Input: part model. Units: mm. Frame: model coordinates. Face numbers are marked on the shaded views. A direction names the side the tool comes from. Round coordinates to 2 decimals unless told otherwise and drop trailing zeros. Loops run counter-clockwise (first coordinate to the right, second up) from the corner with the lowest first, then second, coordinate; pieces in that order, holes last. Notation, with made-up numbers: (-32, -10) -> (25, -10) arc R10 cw to (25, 8) -> close; hole circle Ø7 at (15, 14). An arc over 180 degrees is marked (long way). Answer as a JSON object with one key per item and string values. Group by question number.
Item 1: Section query A-A on y = 0. Return loops of the section in (x, z), and give its area (3 significant figures).
Item 2: Draft query along Z for the marked faces 1, 2, 3 and 4. Return one class per face: released by +Z, released by -Z, zero draft, split by the parting line, or undercut.
Item 3: Pin query (flat end, axial travel): pin 1 (0.9 mm diameter, centred on x = 5, y = -6, fed in from +Z); pin 2 (1.5 mm diameter, centred on x = 6.5, y = 5.5, fed in from -Z); pin 3 (3 mm diameter, centred on x = 6.5, z = -5, fed in from -Y). Return the tip coordinate at first contact, or that it passes through.
Item 4: Section query D-D on y = 3. Return loops of the section in (x, z).
Item 5: Section query C-C on x = 7.75. Return loops of the section in (y, z).
Item 6: Section query B-B on z = 0. Return loops of the section in (x, y), and give its area (3 significant figures).
Item 7: Material intervals for line 1 (Z direction, x = 2.5, y = 0); line 2 (Z direction, x = 1.75, y = 2.5), sorted ascending. Write a range as [from, to].
Item 8: Set-up query: the marked faces 5, 6 and 7. Return all of +Z, -Z, +X, -X, +Y, -Y with unobstructed straight access to the full face (end or side cutting, diameter ignored); none if empty.
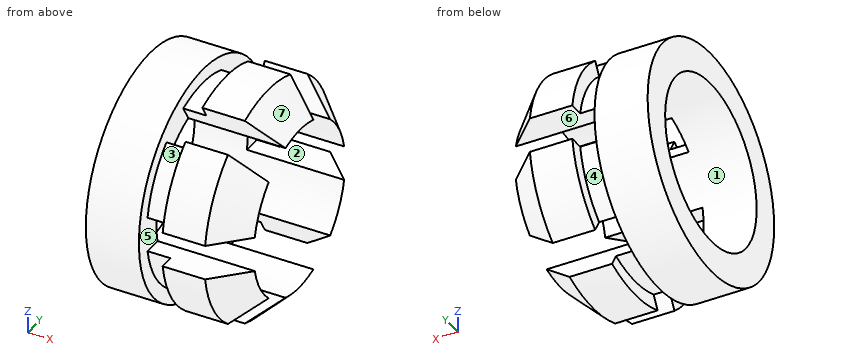
from build123d import *

# Parameters (mm, degrees)
SKETCH_1_R               = 6.5
SKETCH_1_R_2             = 4.7
EXTRUDE_1_DEPTH          = 8.5
SKETCH_2_W               = 1.3
SKETCH_2_H               = 0.8
SKETCH_4_W               = 2
SKETCH_4_H               = 13
CUT_EXTRUDE_1_DEPTH      = 8.5
PATTERN_START            = 3
PATTERN_CIRCULAR_1_DEPTH = 5.5000001


# Read off the part's stored shape, not the designer's step: Круговой массив1
with BuildPart() as part:
    # Эскиз1 → Вытянуть1 (new body)
    with BuildSketch(Plane(origin=(0, 0, 0), x_dir=(0, 0, -1), z_dir=(1, 0, 0))):
        Circle(SKETCH_1_R)
        Circle(SKETCH_1_R_2, mode=Mode.SUBTRACT)
    extrude(amount=EXTRUDE_1_DEPTH)

    # Эскиз2 → Вырез-Повернуть1 (revolve, cut)
    with BuildSketch(Plane.XY, mode=Mode.PRIVATE) as cut_revolve_1_sk:
        with Locations((3.65, 6.1)):
            Rectangle(SKETCH_2_W, SKETCH_2_H)
    revolve(cut_revolve_1_sk.sketch.rotate(Axis((8.5, 0, 0), (-1, 0, 0)), 90), axis=Axis((8.5, 0, 0), (-1, 0, 0)), mode=Mode.SUBTRACT)

    # Эскиз3 → Вырез-Повернуть2 (revolve, cut)
    with BuildSketch(Plane.XY, mode=Mode.PRIVATE) as cut_revolve_2_sk:
        Polygon((8.5, 4.7), (6.7, 6.5), (8.5, 6.5), align=None)
    revolve(cut_revolve_2_sk.sketch.rotate(Axis((8.5, 0, 0), (-1, 0, 0)), 90), axis=Axis((8.5, 0, 0), (-1, 0, 0)), mode=Mode.SUBTRACT)

    # Эскиз4 → Вырез-Вытянуть1 (cut)
    with BuildSketch(Plane(origin=(3, 0, 0), x_dir=(0, 0, -1), z_dir=(1, 0, 0))):
        Rectangle(SKETCH_4_W, SKETCH_4_H)
    extrude(amount=CUT_EXTRUDE_1_DEPTH, mode=Mode.SUBTRACT)

    # Круговой массив1 outline → Круговой массив1 (cut)
    with BuildSketch(Plane.YZ.offset(PATTERN_START)):
        with BuildLine():
            ThreePointArc((3.162217904, -3.477122075), (2.35, -4.070319398), (1.430167097, -4.477122075))
            Line((1.430167097, -4.477122075), (2.345282741, -6.062148865))
            ThreePointArc((2.345282741, -6.062148865), (3.25, -5.629165125), (4.077333548, -5.062148865))
            Line((4.077333548, -5.062148865), (3.162217904, -3.477122075))
        make_face()
        with BuildLine():
            ThreePointArc((-1.430167097, -4.477122075), (-2.35, -4.070319398), (-3.162217904, -3.477122075))
            Line((-3.162217904, -3.477122075), (-4.077333548, -5.062148865))
            ThreePointArc((-4.077333548, -5.062148865), (-3.25, -5.629165125), (-2.345282741, -6.062148865))
            Line((-2.345282741, -6.062148865), (-1.430167097, -4.477122075))
        make_face()
        with BuildLine():
            ThreePointArc((1.430167097, 4.477122075), (2.35, 4.070319398), (3.162217904, 3.477122075))
            Line((3.162217904, 3.477122075), (4.077333548, 5.062148865))
            ThreePointArc((4.077333548, 5.062148865), (3.25, 5.629165125), (2.345282741, 6.062148865))
            Line((2.345282741, 6.062148865), (1.430167097, 4.477122075))
        make_face()
        with BuildLine():
            ThreePointArc((-3.162217904, 3.477122075), (-2.35, 4.070319398), (-1.430167097, 4.477122075))
            Line((-1.430167097, 4.477122075), (-2.345282741, 6.062148865))
            ThreePointArc((-2.345282741, 6.062148865), (-3.25, 5.629165125), (-4.077333548, 5.062148865))
            Line((-4.077333548, 5.062148865), (-3.162217904, 3.477122075))
        make_face()
    extrude(amount=PATTERN_CIRCULAR_1_DEPTH, mode=Mode.SUBTRACT)


solid = part.part
Solved:
{
 "1": {"outline": "(0, -6.5) -> (3, -6.5) -> (3, -5.7) -> (4.3, -5.7) -> (4.3, -6.5) -> (6.7, -6.5) -> (8.5, -4.7) -> (0, -4.7) -> close; (0, 4.7) -> (8.5, 4.7) -> (6.7, 6.5) -> (4.3, 6.5) -> (4.3, 5.7) -> (3, 5.7) -> (3, 6.5) -> (0, 6.5) -> close", "area": "25.3 mm²"},
 "2": {"face 1": "undercut", "face 2": "undercut", "face 3": "released by +Z", "face 4": "released by -Z"},
 "3": {"pin 1": "z = 3.38", "pin 2": "z = -4.44", "pin 3": "y = -5.48"},
 "4": {"outline": "(0, -5.77) -> (3, -5.77) -> (3, -3.62) -> (0, -3.62) -> close; (0, 3.62) -> (3, 3.62) -> (3, 5.77) -> (0, 5.77) -> close"},
 "5": {"outline": "(-5.36, -1) arc R5.45 ccw to (-3.54, -4.14) -> (-3.16, -3.48) arc R4.7 cw to (-4.59, -1) -> close; (-5.36, 1) -> (-4.59, 1) arc R4.7 cw to (-3.16, 3.48) -> (-3.54, 4.14) arc R5.45 ccw to start; (-1.81, -5.14) arc R5.45 ccw to (1.81, -5.14) -> (1.43, -4.48) arc R4.7 cw to (-1.43, -4.48) -> close; (-1.81, 5.14) -> (-1.43, 4.48) arc R4.7 cw to (1.43, 4.48) -> (1.81, 5.14) arc R5.45 ccw to start; (3.16, -3.48) -> (3.54, -4.14) arc R5.45 ccw to (5.36, -1) -> (4.59, -1) arc R4.7 cw to start; (3.16, 3.48) arc R4.7 cw to (4.59, 1) -> (5.36, 1) arc R5.45 ccw to (3.54, 4.14) -> close"},
 "6": {"outline": "(0, -6.5) -> (3, -6.5) -> (3, -4.7) -> (0, -4.7) -> close; (0, 4.7) -> (3, 4.7) -> (3, 6.5) -> (0, 6.5) -> close", "area": "10.8 mm²"},
 "7": {"line 1": "[-6.5, -4.7], [4.7, 6.5]", "line 2": "[-6, -3.98], [3.98, 6]"},
 "8": {"face 5": "none", "face 6": "+X, +Y, -Y", "face 7": "+Z, +X"}
}
